The listing builds one solid part. Answer for the finished solid, in the listing's coordinates (mm). A direction names the side the tool comes from. Coordinates: 2 decimals unless noted, no trailing zeros. Order: outer loops, then holes, each group sorted by start corner. A loop starts at its lowest first (then second) coordinate and runs counter-clockwise, first axis right, second up. Notation, with made-up numbers: (17, 75) -> (54, 75) arc R9 ccw to (54, 87) -> close; hole circle Ø1 at (-8.75, 55). An arc over 180 degrees is marked (long way). Write item = value, one per line.
from build123d import *

# Parameters (mm, degrees)
SKETCH1_W           = 107
SKETCH1_H           = 23.18
BOSS_EXTRUDE1_DEPTH = 39
CUT_EXTRUDE1_DEPTH  = 0.5
CUT_EXTRUDE2_START  = -0.5
CUT_EXTRUDE2_DEPTH  = 0.5
FILLET1_R           = 4
FILLET2_R           = 1
SKETCH5_R           = 2
BOSS_EXTRUDE2_DEPTH = 20
SKETCH7_R           = 2
BOSS_EXTRUDE3_DEPTH = 20


with BuildPart() as part:
    # Sketch1 → Boss-Extrude1 (new body)
    with BuildSketch(Plane(origin=(0, 0, -15), x_dir=(-1, 0, 0), z_dir=(0, 0, -1))):
        with Locations((-15.5, -10.41)):
            Rectangle(SKETCH1_W, SKETCH1_H)
    extrude(amount=-BOSS_EXTRUDE1_DEPTH)

    # Sketch2 → Cut-Extrude1 (cut)
    with BuildSketch(Plane(origin=(69, 0, 0), x_dir=(0, 0, -1), z_dir=(1, 0, 0))):
        with BuildLine():
            Line((-19.125, -9.7175), (-19.125, -11.1025))
            ThreePointArc((-19.125, -11.1025), (-16.781854249, -16.759354249), (-11.125, -19.1025))
            Line((-11.125, -19.1025), (2.125, -19.1025))
            ThreePointArc((2.125, -19.1025), (7.781854249, -16.759354249), (10.125, -11.1025))
            Line((10.125, -11.1025), (10.125, -9.7175))
            ThreePointArc((10.125, -9.7175), (7.781854249, -4.060645751), (2.125, -1.7175))
            Line((2.125, -1.7175), (-11.125, -1.7175))
            ThreePointArc((-11.125, -1.7175), (-16.781854249, -4.060645751), (-19.125, -9.7175))
        make_face()
    extrude(amount=-CUT_EXTRUDE1_DEPTH, mode=Mode.SUBTRACT)

    # Sketch3 → Cut-Extrude2 (cut)
    with BuildSketch(Plane.ZY.offset(38).offset(CUT_EXTRUDE2_START)):
        with BuildLine():
            Line((11.125, -1.7175), (-2.125, -1.7175))
            ThreePointArc((-2.125, -1.7175), (-7.781854249, -4.060645751), (-10.125, -9.7175))
            Line((-10.125, -9.7175), (-10.125, -11.1025))
            ThreePointArc((-10.125, -11.1025), (-7.781854249, -16.759354249), (-2.125, -19.1025))
            Line((-2.125, -19.1025), (11.125, -19.1025))
            ThreePointArc((11.125, -19.1025), (16.781854249, -16.759354249), (19.125, -11.1025))
            Line((19.125, -11.1025), (19.125, -9.7175))
            ThreePointArc((19.125, -9.7175), (16.781854249, -4.060645751), (11.125, -1.7175))
        make_face()
    extrude(amount=CUT_EXTRUDE2_DEPTH, mode=Mode.SUBTRACT)

    # Fillet1
    fillet1_edges = [part.edges().sort_by_distance(p)[0] for p in [
        (-38, -10.41, 24),
        (69, -10.41, 24),
        (-38, -10.41, -15),
        (69, -10.41, -15),
    ]]
    fillet(fillet1_edges, radius=FILLET1_R)

    # Fillet2
    fillet2_edges = [part.edges().sort_by_distance(p)[0] for p in [
        (15.5, -22, -15),
        (15.5, 1.18, -15),
        (-38, 1.18, 4.5),
        (15.5, 1.18, 24),
        (69, 1.18, 4.5),
        (67.828427125, 1.18, 22.828427125),
        (67.828427125, 1.18, -13.828427125),
        (-36.828427125, 1.18, 22.828427125),
        (-36.828427125, 1.18, -13.828427125),
        (-38, -22, 4.5),
        (69, -22, 4.5),
        (15.5, -22, 24),
        (67.828427125, -22, 22.828427125),
        (67.828427125, -22, -13.828427125),
        (-36.828427125, -22, 22.828427125),
        (-36.828427125, -22, -13.828427125),
    ]]
    fillet(fillet2_edges, radius=FILLET2_R)

    # Sketch5 → Boss-Extrude2 (add)
    with BuildSketch(Plane(origin=(69, 0, 0), x_dir=(0, 0, -1), z_dir=(1, 0, 0))):
        with Locations(Location((10.227970674, -5.937982546, 0), (0, 0, 148.897384026))):
            Circle(SKETCH5_R)
    extrude(amount=BOSS_EXTRUDE2_DEPTH)

    # Sketch7 → Boss-Extrude3 (add)
    with BuildSketch(Plane(origin=(68.5, 0, 0), x_dir=(0, 0, -1), z_dir=(1, 0, 0))):
        with Locations(Location((10.325411399, -10.113287546, 0), (0, 0, 100.265525012))):
            Circle(SKETCH7_R)
    extrude(amount=BOSS_EXTRUDE3_DEPTH)


solid = part.part
Q1. The mould has two halves that part along X. Classify faces 1 (the face through (16, -22, 4)), 2 (the face through (68.754, -3.579, -7.255)), 3 (the face through (88.5, -10, -10)): released by +X, released by -X, zero draft, split by the parting line, or undercut.
The answers:
face_1 = zero draft
face_2 = undercut
face_3 = released by +X
Q2. Section B-B, the plane y = -15.5 is taken. Give the vertices of the cut face in (x, z), plus the area to 3 significant figures.
The answers:
outline = (-38, -11) arc R4 ccw to (-34, -15) -> (65, -15) arc R4 ccw to (69, -11) -> (69, -8.81) -> (68.5, -8.81) -> (68.5, 17.81) -> (69, 17.81) -> (69, 20) arc R4 ccw to (65, 24) -> (-34, 24) arc R4 ccw to (-38, 20) -> (-38, 17.81) -> (-37.5, 17.81) -> (-37.5, -8.81) -> (-38, -8.81) -> close
area = 4,130 mm2
Q3. Each of these flat-tipped pins is pushed along its axis until it touches: pin 1 Ø2 at (y, z) = (-6.5, 11.5) entering from +X; pin 2 Ø0.6 at (x, y) = (68.5, -10.5) entering from -Z; pin 3 Ø0.6 at (x, z) = (-37.5, 6.5) entering from +Y; pin 4 Ø1.9 at (y, z) = (-6, -8.5) entering from -X. Where does it stop, or does it pass through?
The answers:
pin_1 = 68.5
pin_2 = -13.4
pin_3 = 1.16
pin_4 = -38
Q4. Find the intervals of material crossed by line 1 along X through (y, z) = (-16.25, -3); line 2 along X through (y, z) = (0, 5); line 3 along Z through (x, y) = (68, -0.5), in increasing order.
The answers:
line_1 = -37.5 to 68.5
line_2 = -38 to 69
line_3 = -13.65 to 22.65
Q5. A tool of negligible diameter and unlimited length cuts with its end or side. For faces 4 (the face through (-36.797, -10.262, 22.859)), 5 (the face through (-37.75, -16.7, -7.84)), 6 (the face through (78.86, -4.33, -9.04)), from which of +Z, -Z, +X, -X, +Y, -Y can it reach the whole face along a straight path? Write none if from no direction.
The answers:
face_4 = +Z, -X, +Y, -Y
face_5 = -X
face_6 = +X
Q6. Section A-A, the plane z = 3 is taken. Give the vertices of the cut face in (x, y).
The answers:
outline = (-38, -21) arc R1 ccw to (-37, -22) -> (68, -22) arc R1 ccw to (69, -21) -> (69, -19.1) -> (68.5, -19.1) -> (68.5, -1.72) -> (69, -1.72) -> (69, 0.18) arc R1 ccw to (68, 1.18) -> (-37, 1.18) arc R1 ccw to (-38, 0.18) -> (-38, -1.72) -> (-37.5, -1.72) -> (-37.5, -19.1) -> (-38, -19.1) -> close
